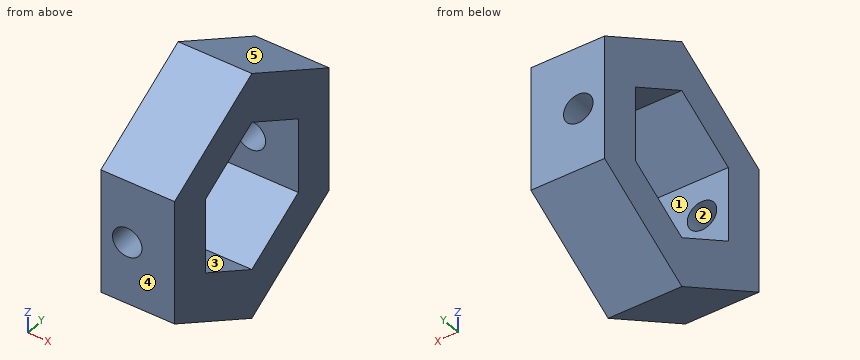
```python
from build123d import *

# Parameters (mm, degrees)
SKETCH214_R     = 1.4
PAD127050_DEPTH = 15
PAD127042_DEPTH = 7


with BuildPart() as pad127050:
    # Sketch214 → Pad127050 (new body, symmetric)
    with BuildSketch(Plane(origin=(75, 0, 0), x_dir=(1, 0, 0), z_dir=(0, -1, 0))):
        with Locations((-22.5, 0)):
            Circle(SKETCH214_R)
    extrude(amount=PAD127050_DEPTH, both=True)


with BuildPart() as wheelcollar:
    # Sketch206 → Pad127042 (new body)
    with BuildSketch(Plane.YZ.offset(57)):
        Polygon((0, 12), (-10.392305, 6), (-10.392305, -6), (0, -12), (10.392305, -6), (10.392305, 6), align=None)
        Polygon((6.25, 3.608439), (0, 7.216878), (-6.25, 3.608439), (-6.25, -3.608439), (0, -7.216878), (6.25, -3.608439), align=None, mode=Mode.SUBTRACT)
    extrude(amount=-PAD127042_DEPTH)

    # Cut007019027: cut Pad127050
    add(pad127050.part, mode=Mode.SUBTRACT)


solid = wheelcollar.part
```
Design review of the part built by this model. Coordinates are the model's own, in mm. Face numbers are marked on the shaded views. A direction names the side the tool comes from. Give positions to 0.01 mm unless a question says otherwise; leave off trailing zeros. Order: outer loops, then holes, each group sorted by start corner. A loop starts at its lowest first (then second) coordinate and runs counter-clockwise, first axis right, second up. Notation, with made-up numbers: (61, 42) -> (76, 42) arc R13 cw to (76, 46) -> close; hole circle Ø5 at (61.5, 48.25). An arc over 180 degrees is marked (long way). Write each question's results on one line, items separated by ' | '. Start each with the question number.
Q1. For pin 1 (2 mm diameter, centred on x = 53, z = -1, fed in from +Y), flat-tipped, find the tip position at first contact; note if it passes through.
Q2. Add section D-D on y = 1.5. Give the boundary of the cut face in (x, z).
Q3. Wall thickness on L1, parallel to Y at x = 56, z = -2.5; L2, parallel to Y at x = 52.5, z = -7; L3, parallel to Z at x = 51, y = 2: over which ranges is each line inside the solid? List them lowest first. Write a range as from..to.
Q4. Add section C-C on x = 52.5. Give the boundary of the cut face in (y, z), and give its area (3 significant figures).
Q5. Mouldability with a two-part tool opening along Z and no side actions: class the marked faces 3, 4 and 5 as +Z half, -Z half, draft (parallel to the pull), parting line (faces both ways), or undercut.
Q6. Machinability: for the marked faces 1 and 2, which of the approach directions +Z, -Z, +X, -X, +Y, -Y give a long, thin tool a straight path to every point of the face, cutting with its end or side? Answer none if there is none.
Q7. Add section B-B on x = 55.5. Give the boundary of the cut face in (y, z), and give its area (3 significant figures).
Q8. Add section A-A on z = 0. Give the boundary of the cut face in (x, y).
Found:
1) pin 1: stops at y = 10.39
2) outline: (50, -11.13) -> (57, -11.13) -> (57, -6.35) -> (50, -6.35) -> close; (50, 6.35) -> (57, 6.35) -> (57, 11.13) -> (50, 11.13) -> close
3) L1: y = -10.39..-6.25, 6.25..10.39 | L2: y = -8.66..-0.38, 0.38..8.66 | L3: z = -10.85..-6.06, 6.06..10.85
4) outline: (-10.39, -6) -> (0, -12) -> (10.39, -6) -> (10.39, -1.4) -> (6.25, -1.4) -> (6.25, -3.61) -> (0, -7.22) -> (-6.25, -3.61) -> (-6.25, -1.4) -> (-10.39, -1.4) -> close; (-10.39, 1.4) -> (-6.25, 1.4) -> (-6.25, 3.61) -> (0, 7.22) -> (6.25, 3.61) -> (6.25, 1.4) -> (10.39, 1.4) -> (10.39, 6) -> (0, 12) -> (-10.39, 6) -> close | area: 216 mm2
5) face 3: undercut | face 4: draft | face 5: +Z half
6) face 1: +X, -X | face 2: +Y, -Y
7) outline: (-10.39, -6) -> (0, -12) -> (10.39, -6) -> (10.39, 6) -> (0, 12) -> (-10.39, 6) -> close; hole (-6.25, -3.61) -> (0, -7.22) -> (6.25, -3.61) -> (6.25, 3.61) -> (0, 7.22) -> (-6.25, 3.61) -> close | area: 239 mm2
8) outline: (50, -10.39) -> (51.1, -10.39) -> (51.1, -6.25) -> (50, -6.25) -> close; (50, 6.25) -> (51.1, 6.25) -> (51.1, 10.39) -> (50, 10.39) -> close; (53.9, -10.39) -> (57, -10.39) -> (57, -6.25) -> (53.9, -6.25) -> close; (53.9, 6.25) -> (57, 6.25) -> (57, 10.39) -> (53.9, 10.39) -> close
